```python
from build123d import *

# Parameters (mm, degrees)
SKETCH2_W           = 156.4
SKETCH2_H           = 55
BOSS_EXTRUDE1_DEPTH = 3.175
SKETCH5_R           = 1.6
CUT_EXTRUDE3_DEPTH  = 83.955232656
SKETCH6_R           = 1.6
CUT_EXTRUDE4_DEPTH  = 83.955232656
SKETCH7_W           = 20
SKETCH7_H           = 20
CUT_EXTRUDE5_DEPTH  = 83.955232656
FILLET1_R           = 5


with BuildPart() as part:
    # Sketch2 → Boss-Extrude1 (new body)
    with BuildSketch(Plane(origin=(0, 0, 0), x_dir=(1, 0, 0), z_dir=(0, 1, 0))):
        Rectangle(SKETCH2_W, SKETCH2_H)
    extrude(amount=BOSS_EXTRUDE1_DEPTH)

    # Sketch5 → Cut-Extrude3 (cut, through all)
    with BuildSketch(Plane(origin=(0, 3.175, 0), x_dir=(1, 0, 0), z_dir=(0, 1, 0))):
        with Locations(Location((-71.2, -23.5, 0), (0, 0, 270))):
            Circle(SKETCH5_R)
        with Locations(Location((-71.258884374, 23.517459766, 0), (0, 0, 90))):
            Circle(SKETCH5_R)
        with Locations(Location((71.258884374, 23.517459766, 0), (0, 0, 270))):
            Circle(SKETCH5_R)
        with Locations(Location((71.2, -23.5, 0), (0, 0, 90))):
            Circle(SKETCH5_R)
    extrude(amount=-CUT_EXTRUDE3_DEPTH, mode=Mode.SUBTRACT)

    # Sketch6 → Cut-Extrude4 (cut, through all)
    with BuildSketch(Plane(origin=(0, 3.175, 0), x_dir=(1, 0, 0), z_dir=(0, 1, 0))):
        with Locations(Location((69.8, -15.6, 0), (0, 0, 270))):
            Circle(SKETCH6_R)
        with Locations(Location((63.4, -15.6, 0), (0, 0, 270))):
            Circle(SKETCH6_R)
        with Locations(Location((57, -15.6, 0), (0, 0, 270))):
            Circle(SKETCH6_R)
        with Locations(Location((50.6, -15.6, 0), (0, 0, 270))):
            Circle(SKETCH6_R)
        with Locations(Location((37.8, -15.6, 0), (0, 0, 270))):
            Circle(SKETCH6_R)
        with Locations(Location((31.4, -15.6, 0), (0, 0, 270))):
            Circle(SKETCH6_R)
        with Locations(Location((44.2, -15.6, 0), (0, 0, 270))):
            Circle(SKETCH6_R)
        with Locations(Location((31.4, 15.6, 0), (0, 0, 90))):
            Circle(SKETCH6_R)
        with Locations(Location((37.8, 15.6, 0), (0, 0, 90))):
            Circle(SKETCH6_R)
        with Locations(Location((44.2, 15.6, 0), (0, 0, 90))):
            Circle(SKETCH6_R)
        with Locations(Location((50.6, 15.6, 0), (0, 0, 90))):
            Circle(SKETCH6_R)
        with Locations(Location((57, 15.6, 0), (0, 0, 90))):
            Circle(SKETCH6_R)
        with Locations(Location((63.4, 15.6, 0), (0, 0, 90))):
            Circle(SKETCH6_R)
        with Locations(Location((69.8, 15.6, 0), (0, 0, 90))):
            Circle(SKETCH6_R)
        with Locations(Location((-31.4, 15.6, 0), (0, 0, 270))):
            Circle(SKETCH6_R)
        with Locations(Location((-37.8, 15.6, 0), (0, 0, 270))):
            Circle(SKETCH6_R)
        with Locations(Location((-44.2, 15.6, 0), (0, 0, 270))):
            Circle(SKETCH6_R)
        with Locations(Location((-50.6, 15.6, 0), (0, 0, 270))):
            Circle(SKETCH6_R)
        with Locations(Location((-57, 15.6, 0), (0, 0, 270))):
            Circle(SKETCH6_R)
        with Locations(Location((-63.4, 15.6, 0), (0, 0, 270))):
            Circle(SKETCH6_R)
        with Locations(Location((-69.8, 15.6, 0), (0, 0, 270))):
            Circle(SKETCH6_R)
        with Locations(Location((-31.4, -15.6, 0), (0, 0, 90))):
            Circle(SKETCH6_R)
        with Locations(Location((-37.8, -15.6, 0), (0, 0, 90))):
            Circle(SKETCH6_R)
        with Locations(Location((-44.2, -15.6, 0), (0, 0, 90))):
            Circle(SKETCH6_R)
        with Locations(Location((-50.6, -15.6, 0), (0, 0, 90))):
            Circle(SKETCH6_R)
        with Locations(Location((-57, -15.6, 0), (0, 0, 90))):
            Circle(SKETCH6_R)
        with Locations(Location((-63.4, -15.6, 0), (0, 0, 90))):
            Circle(SKETCH6_R)
        with Locations(Location((-69.8, -15.6, 0), (0, 0, 90))):
            Circle(SKETCH6_R)
    extrude(amount=-CUT_EXTRUDE4_DEPTH, mode=Mode.SUBTRACT)

    # Sketch7 → Cut-Extrude5 (cut, through all)
    with BuildSketch(Plane(origin=(0, 3.175, 0), x_dir=(1, 0, 0), z_dir=(0, 1, 0))):
        Rectangle(SKETCH7_W, SKETCH7_H)
    extrude(amount=-CUT_EXTRUDE5_DEPTH, mode=Mode.SUBTRACT)

    # Fillet1
    fillet1_edges = [part.edges().sort_by_distance(p)[0] for p in [
        (78.2, 1.5875, 27.5),
        (-78.2, 1.5875, 27.5),
        (-78.2, 1.5875, -27.5),
        (78.2, 1.5875, -27.5),
    ]]
    fillet(fillet1_edges, radius=FILLET1_R)


solid = part.part
```
Could you check a few things on this model? Use its own coordinates, in mm. A direction names the side the tool comes from. Round coordinates to 2 decimals unless told otherwise and drop trailing zeros. Loops run counter-clockwise (first coordinate to the right, second up) from the corner with the lowest first, then second, coordinate; pieces in that order, holes last. Notation, with made-up numbers: (49.5, 35) - (56.5, 35) arc R23 ccw to (56.5, 70) - close; hole circle Ø4 at (82.5, 48). An arc over 180 degrees is marked (long way). Answer in a Markdown table with one row per item. Add a question column.
(1) If we section it at C-C (y = 2.5): State how many separate pieces and enclosed holes the cut face has, plus the area to 3 significant figures.
(2) If we mould it in two halves opening along X, with no side actions, what happens to faces 1 (the face through (-1, 3.175, 12)), 2 (the face through (49.25, 1.61, -16.46)), 3 (the face through (-78.2, 2, 0)), 4 (the face through (45.62, 1.61, -16.34))? For each: pulls with the +X half, pulls with the -X half, needs draft (parallel to the pull), parting line crosses it, or undercut.
(3) I need wall thicknesses on line 1 along X through (y, z) = (1.15, -3.5); line 2 along Z through (x, y) = (-69.8, 2.1); line 3 along Z through (x, y) = (32, 2.9). Which ranges of each line are inside material? Lowest first, please.
(4) If we section it at B-B (x = 63.4): Please give me the cut outline in (y, z) (3 decimals), plus the area to 3 significant figures.
(5) If we section it at A-A (z = 2): Please give me the cut outline in (x, y) (3 decimals), plus the area to 3 significant figures.
(6) I'm going to push a flat-ended pin straight in: pin 1 (1.9 mm diameter, centred on x = -37.8, z = -15.6, fed in from -Y). Where does the tip first touch, or does it pass through?
(7) For faces 5 (the face through (10, 2, 0)), 6 (the face through (76.7, 1.61, -26.07)), which set-ups out of +Z, -Z, +X, -X, +Y, -Y let a thin tool reach every point of the face, with its end or its side?
Model answer:
| question | item | result |
|---|---|---|
| 1 | separate pieces | 1 |
| 1 | enclosed holes | 33 |
| 1 | area | 7,920 mm² |
| 2 | face 1 | needs draft |
| 2 | face 2 | undercut |
| 2 | face 3 | pulls with the -X half |
| 2 | face 4 | undercut |
| 3 | line 1 | x = -78.2 to -10, 10 to 78.2 |
| 3 | line 2 | z = -27.5 to -24.17, -22.86 to -17.2, -14 to 14, 17.2 to 22.73, 24.27 to 27.5 |
| 3 | line 3 | z = -27.5 to -17.08, -14.12 to 14.12, 17.08 to 27.5 |
| 4 | outline | (0, -27.5) - (3.175, -27.5) - (3.175, -17.2) - (0, -17.2) - close; (0, -14) - (3.175, -14) - (3.175, 14) - (0, 14) - close; (0, 17.2) - (3.175, 17.2) - (3.175, 27.5) - (0, 27.5) - close |
| 4 | area | 154 mm² |
| 5 | outline | (-78.2, 0) - (-10, 0) - (-10, 3.175) - (-78.2, 3.175) - close; (10, 0) - (78.2, 0) - (78.2, 3.175) - (10, 3.175) - close |
| 5 | area | 433 mm² |
| 6 | pin 1 | passes through |
| 7 | face 5 | +Y, -Y |
| 7 | face 6 | -Z, +X, +Y, -Y |
